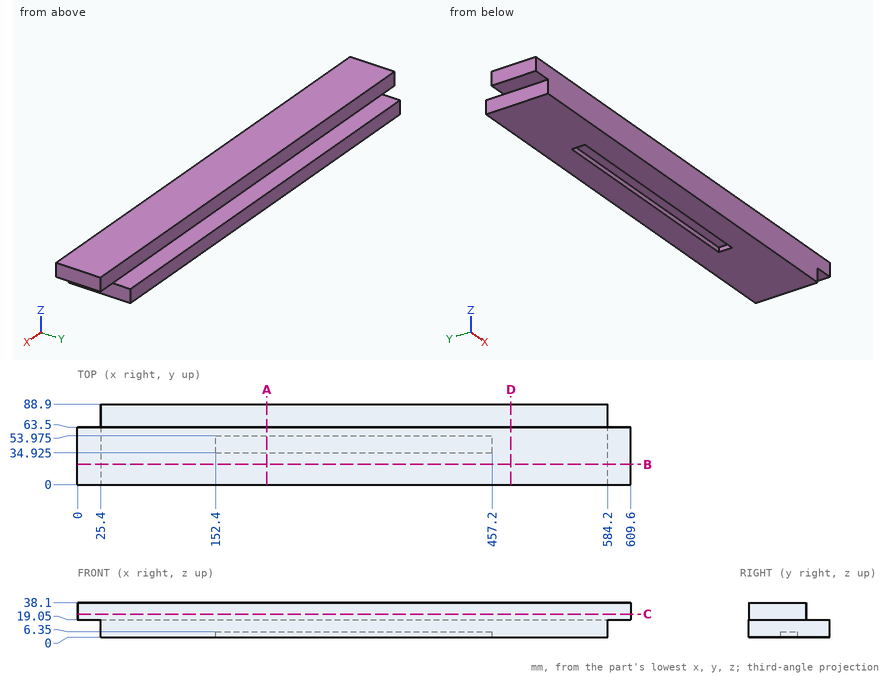
Part print with two shaded views. Sizes in mm from the minimum x, y, z corner. Give positions to 0.01 mm unless a question says otherwise; leave off trailing zeros. Order: outer loops, then holes, each group sorted by start corner. A loop starts at its lowest first (then second) coordinate and runs counter-clockwise, first axis right, second up. Notation, with made-up numbers: M 44,52 L 64,52 A23 ccw 64,69 Z; hole C -6.75,84 d10. An arc over 180 degrees is marked long. Use one line per item in the form item = value.
1) Drop flat-ended pins along their axis: pin 1 (9.5 mm diameter, centred on y = 31.5, z = 5, fed in from +X); pin 2 (20.5 mm diameter, centred on x = 194, y = 74.5, fed in from +Z); pin 3 (5.5 mm diameter, centred on x = 218, z = 30.5, fed in from +Y). Give the stop position or say it passes through.
Calculated:
pin_1 = 584.2
pin_2 = 19.05
pin_3 = 63.5
2) Saw through at B-B (y = 22.5). Give the cut face in (x, z).
Calculated:
outline = M 0,19.05 L 25.4,19.05 L 25.4,0 L 584.2,0 L 584.2,19.05 L 609.6,19.05 L 609.6,38.1 L 0,38.1 Z
3) Saw through at A-A (x = 208.5). Give the cut face in (y, z) (3 decimals).
Calculated:
outline = M 0,0 L 34.925,0 L 34.925,6.35 L 53.975,6.35 L 53.975,0 L 88.9,0 L 88.9,19.05 L 63.5,19.05 L 63.5,38.1 L 0,38.1 Z
4) Probe probe 1 along X at (y, z) = (34.5, 16); probe 2 along Z at (x, y) = (245.5, 70.5); probe 3 along Y at (x, z) = (243, 4.5) (3 decimals). List the from-to ranges inside material, lowest first.
Calculated:
probe_1 = 25.4 to 584.2
probe_2 = 0 to 19.05
probe_3 = 0 to 34.925, 53.975 to 88.9
5) Saw through at C-C (z = 25.5). Give the cut face in (x, y).
Calculated:
outline = M 0,0 L 609.6,0 L 609.6,63.5 L 0,63.5 Z
6) Saw through at D-D (x = 477.5). Give the cut face in (y, z), plus the area to 3 significant figures.
Calculated:
outline = M 0,0 L 88.9,0 L 88.9,19.05 L 63.5,19.05 L 63.5,38.1 L 0,38.1 Z
area = 2,900 mm2
